```python
from build123d import *

# Parameters (mm, degrees)
ESQUISSE2_W        = 304.8
ESQUISSE2_H        = 27.559
BOSS_EXTRU_1_DEPTH = 6.35


with BuildPart() as part:
    # Esquisse2 → Boss.-Extru.1 (new body)
    with BuildSketch(Plane(origin=(0, 0, 0), x_dir=(0, 0, -1), z_dir=(1, 0, 0))):
        Polygon((0, 152.4), (0, 0), (-304.8, 0), (-127, 152.4), align=None)
        with Locations((-152.4, -13.7795)):
            Rectangle(ESQUISSE2_W, ESQUISSE2_H)
    extrude(amount=BOSS_EXTRU_1_DEPTH)


solid = part.part
```
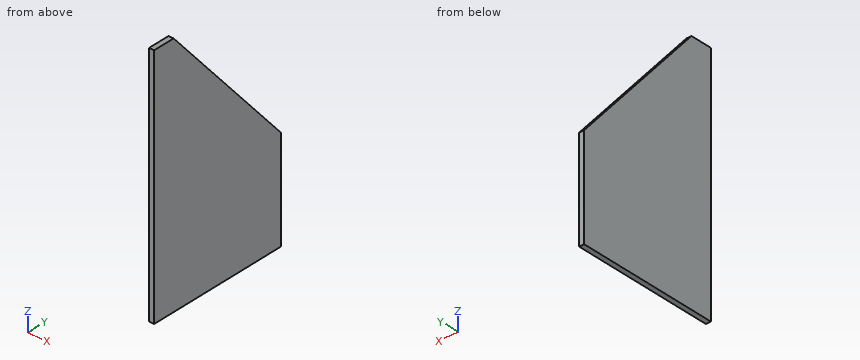
The listing builds one solid part. Answer for the finished solid, in the listing's coordinates (mm). Coordinates: 2 decimals unless noted, no trailing zeros. Write each loop counter-clockwise with the first axis right and the second up, starting at its lowest first coordinate (ties: lowest second). Pieces come first, ordered by that corner, then holes. Notation, with made-up numbers: (67.25, -18.5) - (119.25, -18.5) arc R29 ccw to (119.25, 12.5) - close; hole circle Ø9 at (21.5, 27). An arc over 180 degrees is marked (long way). One line per item, written item: value.
1) Consider line 1 along Z through (x, y) = (5.5, 26.5); line 2 along Y through (x, z) = (5.5, 249); line 3 along Z through (x, y) = (5, 107.5). Determine where each line is inside the solid, lowest interval first. Write a range as from..to.
Geometry check:
line 1: z = 0..273.88
line 2: y = -27.56..47.83
line 3: z = 0..179.38
2) Find section A-A (x = 2.75). Give the vertices of the cut face in (y, z).
Geometry check:
outline: (-27.56, 0) - (152.4, 0) - (152.4, 127) - (0, 304.8) - (-27.56, 304.8) - close
3) Find section C-C (z = 225). Give the vertices of the cut face in (x, y), and give its area (3 significant figures).
Geometry check:
outline: (0, -27.56) - (6.35, -27.56) - (6.35, 68.4) - (0, 68.4) - close
area: 609 mm2
4) Find section B-B (y = 27). Give the vertices of the cut face in (x, z).
Geometry check:
outline: (0, 0) - (6.35, 0) - (6.35, 273.3) - (0, 273.3) - close
